from build123d import *

# Parameters (mm, degrees)
BOSS_EXTRUDE1_DEPTH = 59
BOSS_EXTRUDE6_DEPTH = 12.75
SKETCH3_14_R        = 1.75
CUT_EXTRUDE3_DEPTH  = 12.75


with BuildPart() as part:
    # Sketch1 → Boss-Extrude1 (new body)
    with BuildSketch(Plane.XY):
        Polygon((0, 8), (0, 18), (-10, 18), (-38, -10), (0, -10), (0, 0), (-6.5, -3.75277675), (-6.5, 11.75277675), align=None)
    extrude(amount=BOSS_EXTRUDE1_DEPTH)

    # Sketch3 → Boss-Extrude6 (add)
    with BuildSketch(Plane.XZ.offset(10)):
        with BuildLine():
            Line((-25.25, 48.75), (-25.25, 39.25))
            Line((-25.25, 39.25), (-30, 39.25))
            ThreePointArc((-30, 39.25), (-34.75, 44), (-30, 48.75))
            Line((-30, 48.75), (-25.25, 48.75))
        make_face()
    boss_extrude6 = extrude(amount=-BOSS_EXTRUDE6_DEPTH)

    # Sketch3<14> → Cut-Extrude3 (cut)
    with BuildSketch(Plane.XZ.offset(10)):
        with Locations((-30, 44)):
            Circle(SKETCH3_14_R)
    cut_extrude3 = extrude(amount=-CUT_EXTRUDE3_DEPTH, mode=Mode.SUBTRACT)

    # Mirror1: Boss-Extrude6, Cut-Extrude3 across plane
    add(boss_extrude6.mirror(Plane.XY.offset(29.5)))
    add(cut_extrude3.mirror(Plane.XY.offset(29.5)), mode=Mode.SUBTRACT)


solid = part.part
Source: CAD feature listing. Evaluate the final solid. Frame: model axes, mm. A direction names the side the tool comes from. Round coordinates to 2 decimals unless told otherwise and drop trailing zeros. Loops run counter-clockwise (first coordinate to the right, second up) from the corner with the lowest first, then second, coordinate; pieces in that order, holes last. Notation, with made-up numbers: (13.25, 43.25) - (38.25, 43.25) arc R28 ccw to (38.25, 77.25) - close; hole circle Ø2 at (37.5, 12.5). An arc over 180 degrees is marked (long way). Write item = value, one per line. Start each with the question number.
Item 1: Section query D-D on z = 11. Output: boundary loops of the cut face in (x, y).
Item 2: Section query A-A on z = 44. Output: boundary loops of the cut face in (x, y).
Item 3: Reachability of faces 5 (the face through (-29, 1, 19.75)), 6 (the face through (-29, 1, 10.25)), 7 (the face through (-28, 2.75, 15)), 8 (the face through (-3.295, 9.903, 29.087)) from +Z, -Z, +X, -X, +Y, -Y: full face, straight path, thin tool, end or side. Return the list, or none.
Item 4: Mould query, pull axis Z, two halves, no side actions, for faces 1 (the face through (-34.75, -1.01, 15.1)), 2 (the face through (0, -5, 29)), 3 (the face through (-29, 1, 48.75)), 4 (the face through (-31.29, -3.71, 13.82)). Classes: released by +Z, released by -Z, zero draft, split by the parting line, or undercut.
Item 5: First-contact query: pin 1 Ø10.5 at (x, z) = (-28.5, 13.5) entering from +Y; pin 2 Ø10.5 at (x, z) = (-30, 42) entering from +Y; pin 3 Ø12 at (y, z) = (12.5, 48) entering from -X. Flat tips, straight axial feed; report the tip coordinate or a pass-through.
Item 6: Section query C-C on x = -27.5. Output: boundary loops of the cut face in (y, z), plus the area to 3 significant figures.
Item 7: Section query B-B on y = 1. Output: boundary loops of the cut face in (x, z).
Item 8: Material intervals for line 1 (Z direction, x = -30, y = -1.5); line 2 (Z direction, x = -30, y = -7); line 3 (X direction, y = -2.25, z = 15), sorted ascending.
Results list:
q1.outline = (-38, -10) - (0, -10) - (0, 0) - (-6.5, -3.75) - (-6.5, 11.75) - (0, 8) - (0, 18) - (-10, 18) - (-25.25, 2.75) - (-32.56, 2.75) - (-32.56, -4.56) - close
q2.outline = (-38, -10) - (-31.75, -10) - (-31.75, 2.75) - (-34.75, 2.75) - (-34.75, -6.75) - close; (-28.25, -10) - (0, -10) - (0, 0) - (-6.5, -3.75) - (-6.5, 11.75) - (0, 8) - (0, 18) - (-10, 18) - (-25.25, 2.75) - (-28.25, 2.75) - close
q3.face_5 = -X, +Y
q3.face_6 = -Z, -X, +Y
q3.face_7 = +Z, -Z, -X, +Y
q3.face_8 = +Z, -Z
q4.face_1 = undercut
q4.face_2 = zero draft
q4.face_3 = released by +Z
q4.face_4 = undercut
q5.pin_1 = 4.75
q5.pin_2 = 3.25
q5.pin_3 = -21.5
q6.outline = (-10, 0) - (0.5, 0) - (0.5, 10.25) - (2.75, 10.25) - (2.75, 19.75) - (0.5, 19.75) - (0.5, 39.25) - (2.75, 39.25) - (2.75, 48.75) - (0.5, 48.75) - (0.5, 59) - (-10, 59) - close
q6.area = 662 mm²
q7.outline = (-30, 10.25) - (-27, 10.25) - (-27, 0) - (-6.5, 0) - (-6.5, 59) - (-27, 59) - (-27, 48.75) - (-30, 48.75) arc R4.75 ccw to (-30, 39.25) - (-27, 39.25) - (-27, 19.75) - (-30, 19.75) arc R4.75 ccw to start; hole circle Ø3.5 at (-30, 15); hole circle Ø3.5 at (-30, 44)
q8.line_1 = 10.25 to 13.25, 16.75 to 19.75, 39.25 to 42.25, 45.75 to 48.75
q8.line_2 = 0 to 13.25, 16.75 to 42.25, 45.75 to 59
q8.line_3 = -34.75 to -31.75, -28.25 to -6.5, -3.9 to 0
